Geometry check sheet. Reference: the model listing, model coordinates, mm. A direction names the side the tool comes from. Give positions to 0.01 mm unless a question says otherwise; leave off trailing zeros. Loops run counter-clockwise (first coordinate to the right, second up) from the corner with the lowest first, then second, coordinate; pieces in that order, holes last. Notation, with made-up numbers: (47, -14) -> (60, -14) arc R7 cw to (60, -7) -> close; hole circle Ø8 at (74.5, -33.5). An arc over 180 degrees is marked (long way). Write each question's results on one line, items separated by ' | '. Start each with the question number.
1) Sectioned sample at A-A on x = 7. Record the cut outline in (y, z), then the cut area to 3 significant figures.
2) Sectioned sample at C-C on x = 10.5. Record the cut outline in (y, z), then the cut area to 3 significant figures.
3) Scan lines: line 1 (X direction, y = 7.5, z = 1.95); line 2 (Y direction, x = 7, z = 2.35); line 3 (Y direction, x = 7, z = 6.55). Record each from-to range of solid material in increasing order. Write a range as from..to.
4) Sectioned sample at B-B on z = 6. Record the cut outline in (x, y), then the cut area to 3 significant figures.
5) Draft check along X on faces 3 (the face through (7, 15, 4)), 4 (the face through (14, 7, 4)), 5 (the face through (8.18, 5.24, 5.54)). Enter one of: pulls with the +X half, pulls with the -X half, needs draft (parallel to the pull), parting line crosses it, or undercut.
6) Depth check by flat-ended pin: pin 1 (8 mm diameter, centred on x = 8.5, y = 6.5, fed in from +Z); pin 2 (1.5 mm diameter, centred on x = 8, y = 8, fed in from +Z). Enter the tip coordinate at first touch or a pass-through.
7) Set-up check for faces 1 (the face through (8, 6, 3)), 2 (the face through (6.9, 2.3, 5.8)): record each of +Z, -Z, +X, -X, +Y, -Y from which the full face is reachable in a straight line by a thin tool's end or side.
8) Sectioned sample at D-D on y = 3. Record the cut outline in (x, z), then the cut area to 3 significant figures.
```python
from build123d import *

# Parameters (mm, degrees)
SKETCH_W        = 14
SKETCH_H        = 15
PAD_DEPTH       = 8
SKETCH001_R     = 1.5
POCKET_DEPTH    = 8.001
SKETCH002_R     = 2.55
POCKET001_DEPTH = 5
CHAMFER_SIZE    = 4.5


with BuildPart() as part:
    # Sketch → Pad (new body)
    with BuildSketch(Plane.XY):
        with Locations((7, 7.5)):
            Rectangle(SKETCH_W, SKETCH_H)
    extrude(amount=PAD_DEPTH)

    # Sketch001 (on Face5 of Pad) → Pocket (cut, through all)
    with BuildSketch(Plane(origin=(0, 0, 0), x_dir=(1, 0, 0), z_dir=(0, 0, -1))):
        with Locations((7, -7.5)):
            Circle(SKETCH001_R)
    extrude(amount=-POCKET_DEPTH, mode=Mode.SUBTRACT)

    # Sketch002 (on Face5 of Pocket) → Pocket001 (cut)
    with BuildSketch(Plane.XY.offset(8)):
        with Locations((7, 7.5)):
            Circle(SKETCH002_R)
    extrude(amount=-POCKET001_DEPTH, mode=Mode.SUBTRACT)

    # Chamfer
    chamfer_edges = [part.edges().sort_by_distance(p)[0] for p in [
        (7, 0, 8),
    ]]
    chamfer(chamfer_edges, length=CHAMFER_SIZE)


solid = part.part
```
Result:
1) outline: (0, 0) -> (6, 0) -> (6, 3) -> (4.95, 3) -> (4.95, 8) -> (4.5, 8) -> (0, 3.5) -> close; (9, 0) -> (15, 0) -> (15, 8) -> (10.05, 8) -> (10.05, 3) -> (9, 3) -> close | area: 75.4 mm^2
2) outline: (0, 0) -> (15, 0) -> (15, 8) -> (4.5, 8) -> (0, 3.5) -> close | area: 110 mm^2
3) line 1: 0..5.5, 8.5..14 | line 2: 0..6, 9..15 | line 3: 3.05..4.95, 10.05..15
4) outline: (0, 2.5) -> (14, 2.5) -> (14, 15) -> (0, 15) -> close; hole circle Ø5.1 at (7, 7.5) | area: 155 mm^2
5) face 3: needs draft | face 4: pulls with the +X half | face 5: undercut
6) pin 1: z = 8 | pin 2: z = 3
7) face 1: +Z | face 2: +Z, +X, -X, -Y
8) outline: (0, 0) -> (14, 0) -> (14, 6.5) -> (0, 6.5) -> close | area: 91.0 mm^2
